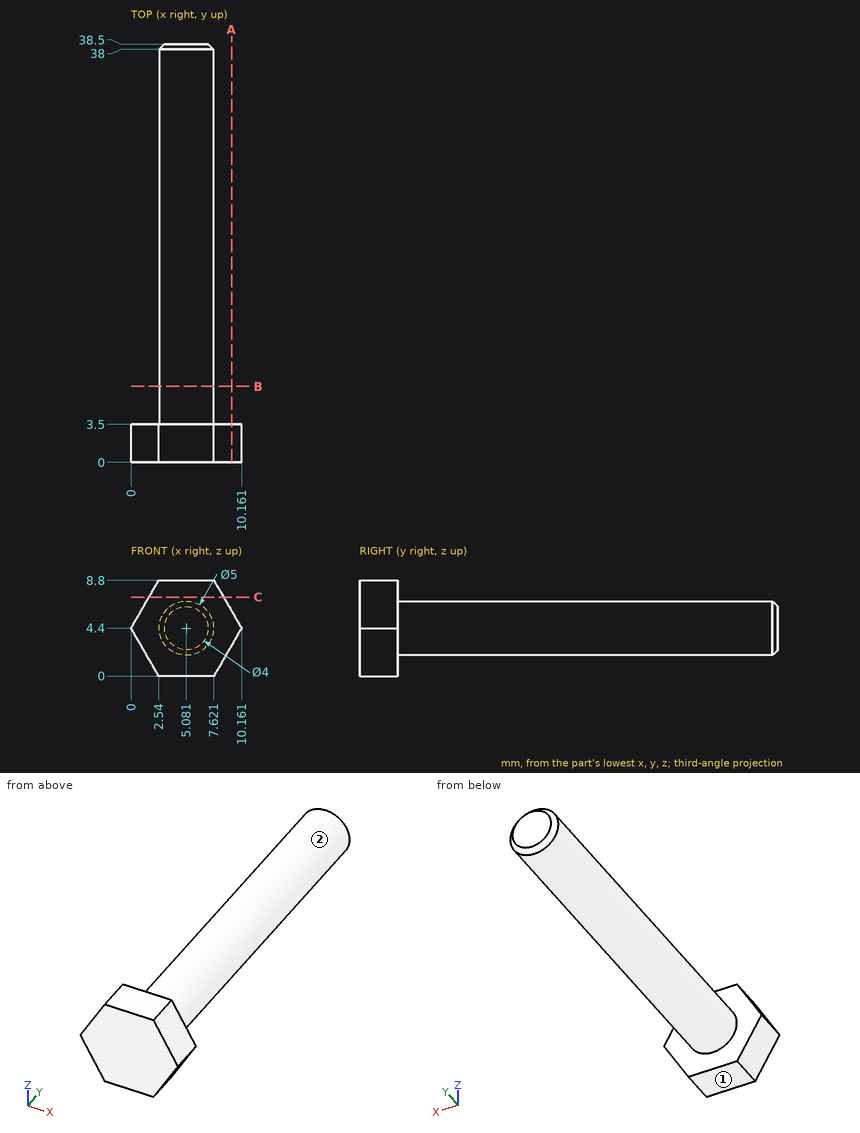
Check sheet for the drawn part. Datum: minimum x, y, z corner. Units: mm. A direction names the side the tool comes from. Round coordinates to 2 decimals unless told otherwise and drop trailing zeros. Order: outer loops, then holes, each group sorted by start corner. A loop starts at its lowest first (then second) coordinate and runs counter-clockwise, first axis right, second up. Notation, with made-up numbers: M 82.25,-0.5 L 98.25,-0.5 A15 ccw 98.25,18.5 Z; hole C 38,28.5 d3. An arc over 180 degrees is marked long. Write each question's results on one line, items separated by ' | '. Start each with the question number.
1. Set-up check for the marked faces 1 and 2: record each of +Z, -Z, +X, -X, +Y, -Y from which the full face is reachable in a straight line by a thin tool's end or side.
2. Material ranges on L1, parallel to Y at x = 6.75, z = 1.75; L2, parallel to Z at x = 5.25, y = 18 (1 decimal); L3, parallel to Z at x = 6.75, y = 30, recorded low to high. Write a range as from..to.
3. Cross-section at C-C on z = 7.25. Record the boundary of the cut face in (x, y) (1 decimal).
4. Cross-section at B-B on y = 7. Record the boundary of the cut face in (x, z), plus the area to 3 significant figures.
5. Cross-section at A-A on x = 9.25. Record the boundary of the cut face in (y, z).
6. Go/stop test with flat-tipped pins: P1, Ø4, axis at x = 7, y = 29, coming from the -Z side; P2, Ø5, axis at y = 21, z = 2, coming from the -X side; P3, Ø1.5, axis at x = 8.5, y = 5.5, coming from the -Z side; P4, Ø3, axis at x = 6.5, y = 11.5, coming from the +Z side. Record where each tip stops, or that it passes through.
Resolved:
1) face 1: -Z, +X, -X, +Y, -Y | face 2: +Y
2) L1: 0..3.5 | L2: 1.9..6.9 | L3: 2.54..6.26
3) outline: M 1.6,0 L 8.5,0 L 8.5,3.5 L 1.6,3.5 Z
4) outline: C 5.08,4.4 d5 | area: 19.6 mm2
5) outline: M 0,2.82 L 3.5,2.82 L 3.5,5.98 L 0,5.98 Z
6) P1: z = 1.9 | P2: x = 2.58 | P3: through | P4: z = 6.9
